Part model, mm, in its own coordinate system. A direction names the side the tool comes from. Round coordinates to 2 decimals unless told otherwise and drop trailing zeros. Write each loop counter-clockwise with the first axis right and the second up, starting at its lowest first coordinate (ties: lowest second). Pieces come first, ordered by that corner, then holes. Notation, with made-up numbers: M -3,-13.75 L 9,-13.75 A34 cw 9,19.25 Z; hole C 25.25,25.25 d9. An arc over 180 degrees is marked long. Answer as a JSON object with one key per item and string values. Group by question number.
1. Band-saw the part on C-C, the plane z = 22.5. Write the cut outline in (x, y), plus the area to 3 significant figures.
2. Band-saw the part on B-B, the plane z = -11. Write the cut outline in (x, y).
3. Band-saw the part on D-D, the plane x = 3.5. Write the cut outline in (y, z).
4. Drill centre lines: line 1 (X direction, y = 1.45, z = -22.5); line 2 (X direction, y = 1, z = 22). Where is each one in solid material? Low to high. Write a range as from..to.
5. Which spindle directions (+Z, -Z, +X, -X, +Y, -Y) get a long thin tool onto all of the face, cutting with end or side? Do faces 1 (the face through (-13, 2, 12)), 2 (the face through (27.5, 1, 0)). Say none if no direction does.
6. Two-plate mould, pull along X, no slides. Class faces 3 (the face through (-27.5, 1, 0)), 4 (the face through (-11, 30, 7)), 5 (the face through (-0.33, 22.48, 13.36)), 6 (the face through (23.51, 0.99, 21.39)): +X half, -X half, draft (parallel to the pull), parting line (faces both ways), or undercut.
7. Band-saw the part on A-A, the plane x = 22.5. Write the cut outline in (y, z), plus the area to 3 significant figures.
8. Drop flat-ended pins along their axis: pin 1 (1.8 mm diameter, centred on x = -22.5, z = -22.5, fed in from +Y); pin 2 (5 mm diameter, centred on x = -21.5, z = 21, fed in from +Y); pin 3 (1 mm diameter, centred on y = 4, z = -7, fed in from -X); pin 4 (10 mm diameter, centred on x = 18, y = 16, fed in from -Z). Give the stop position or say it passes through.
from build123d import *

# Parameters (mm, degrees)
SKETCH_1_W               = 55
SKETCH_1_H               = 55
SKETCH_1_R               = 12.5
EXTRUDE_1_DEPTH          = 2
SKETCH_2_R               = 14.5
SKETCH_2_R_2             = 12.5
EXTRUDE_1_2_DEPTH        = 30
CUT_EXTRUDE_1_DEPTH      = 50.117206761
CUT_EXTRUDE_1_DEPTH_BACK = 50.117206761
SKETCH_3_R               = 2.5
CUT_EXTRUDE_7_DEPTH      = 50.117206822
CUT_EXTRUDE_7_DEPTH_BACK = 50.117206822
SKETCH_4_R               = 1.5


with BuildPart() as part:
    # Эскиз1 → Extrude 1 (new body)
    with BuildSketch(Plane(origin=(0, 0, 0), x_dir=(1, 0, 0), z_dir=(0, 1, 0))):
        Rectangle(SKETCH_1_W, SKETCH_1_H)
        with Locations(Location((0, 0, 0), (0, 0, 270))):
            Circle(SKETCH_1_R, mode=Mode.SUBTRACT)
    extrude(amount=EXTRUDE_1_DEPTH)

    # Эскиз2 → Extrude 1 2 (add)
    with BuildSketch(Plane.XZ):
        Circle(SKETCH_2_R)
        Circle(SKETCH_2_R_2, mode=Mode.SUBTRACT)
    extrude(amount=-EXTRUDE_1_2_DEPTH)

    # Эскиз3 → Вырез-Вытянуть1 (cut, two sides: drawn at the far end of the back side and taken through both)
    with BuildSketch(Plane.XY.offset(-CUT_EXTRUDE_1_DEPTH_BACK)):
        with Locations((0, 20)):
            Circle(SKETCH_3_R)
    extrude(amount=CUT_EXTRUDE_1_DEPTH + CUT_EXTRUDE_1_DEPTH_BACK, mode=Mode.SUBTRACT)

    # Эскиз4 → Вырез-Вытянуть7 (cut, two sides: drawn at the far end of the back side and taken through both)
    with BuildSketch(Plane(origin=(0, 0, 0), x_dir=(1, 0, 0), z_dir=(0, 1, 0)).offset(-CUT_EXTRUDE_7_DEPTH_BACK)):
        with Locations(Location((-22.5, 22.5, 0), (0, 0, 270))):
            Circle(SKETCH_4_R)
        with Locations(Location((22.5, 22.5, 0), (0, 0, 270))):
            Circle(SKETCH_4_R)
        with Locations(Location((22.5, -22.5, 0), (0, 0, 270))):
            Circle(SKETCH_4_R)
        with Locations(Location((-22.5, -22.5, 0), (0, 0, 270))):
            Circle(SKETCH_4_R)
    extrude(amount=CUT_EXTRUDE_7_DEPTH + CUT_EXTRUDE_7_DEPTH_BACK, mode=Mode.SUBTRACT)


solid = part.part
Worked answers:
{
 "1": {"outline": "M -27.5,0 L -24,0 L -24,2 L -27.5,2 Z; M -21,0 L 21,0 L 21,2 L -21,2 Z; M 24,0 L 27.5,0 L 27.5,2 L 24,2 Z", "area": "98.0 mm^2"},
 "2": {"outline": "M -27.5,0 L -5.94,0 L -5.94,30 L -9.45,30 L -9.45,2 L -27.5,2 Z; M 5.94,0 L 27.5,0 L 27.5,2 L 9.45,2 L 9.45,30 L 5.94,30 Z"},
 "3": {"outline": "M 0,-27.5 L 2,-27.5 L 2,-14.07 L 30,-14.07 L 30,-12 L 0,-12 Z; M 0,12 L 30,12 L 30,14.07 L 2,14.07 L 2,27.5 L 0,27.5 Z"},
 "4": {"line 1": "x = -27.5..-24, -21..21, 24..27.5", "line 2": "x = -27.5..-23.91, -21.09..21.09, 23.91..27.5"},
 "5": {"face 1": "+Y", "face 2": "+Z, -Z, +X, +Y, -Y"},
 "6": {"face 3": "-X half", "face 4": "draft", "face 5": "undercut", "face 6": "undercut"},
 "7": {"outline": "M 0,-27.5 L 2,-27.5 L 2,-24 L 0,-24 Z; M 0,-21 L 2,-21 L 2,21 L 0,21 Z; M 0,24 L 2,24 L 2,27.5 L 0,27.5 Z", "area": "98.0 mm^2"},
 "8": {"pin 1": "passes through", "pin 2": "stops at y = 2", "pin 3": "stops at x = -12.96", "pin 4": "stops at z = -6.42"}
}
